Check sheet for the modelled part. Datum: model origin and axes. Units: mm. A direction names the side the tool comes from. Coordinates: 2 decimals unless noted, no trailing zeros. Write each loop counter-clockwise with the first axis right and the second up, starting at its lowest first coordinate (ties: lowest second). Pieces come first, ordered by that corner, then holes. Notation, with made-up numbers: (23.25, 1) -> (75.25, 1) arc R23 cw to (75.25, 18) -> close; hole circle Ø1 at (68.5, 22). An arc over 180 degrees is marked (long way). Put each result on its own line as item: value.
```python
from build123d import *

# Parameters (mm, degrees)
SKETCH1_W                = 25.4
SKETCH1_H                = 50.8
SKETCH1_W_2              = 19.05
SKETCH1_H_2              = 44.45
BOSS_EXTRUDE1_DEPTH      = 342.9
CUT_EXTRUDE1_DEPTH       = 1
CUT_EXTRUDE1_DEPTH_BACK  = 26.4
CUT_EXTRUDE2_REACH       = 27.4
SKETCH3_R                = 11.1125
M3_CLEARANCE_HOLE1_D     = 3.4
M3_CLEARANCE_HOLE1_DEPTH = 3.175
SKETCH9_R                = 4.5
CUT_EXTRUDE3_DEPTH       = 12.7


with BuildPart() as part:
    # Sketch1 → Boss-Extrude1 (new body, symmetric)
    with BuildSketch(Plane(origin=(0, 0, 0), x_dir=(0, 0, -1), z_dir=(1, 0, 0))):
        Rectangle(SKETCH1_W, SKETCH1_H)
        Rectangle(SKETCH1_W_2, SKETCH1_H_2, mode=Mode.SUBTRACT)
    extrude(amount=BOSS_EXTRUDE1_DEPTH, both=True)

    # Sketch2 → Cut-Extrude1 (cut, two sides)
    with BuildSketch(Plane(origin=(0, 0, -12.7), x_dir=(-1, 0, 0), z_dir=(0, 0, -1))) as cut_extrude1_sk:
        Polygon((342.9, -25.4), (342.9, 25.4), (313.570606325, -25.4), align=None)
        Polygon((-342.9, -25.4), (-313.570606325, -25.4), (-342.9, 25.4), align=None)
    extrude(amount=CUT_EXTRUDE1_DEPTH, mode=Mode.SUBTRACT)
    extrude(cut_extrude1_sk.sketch, amount=-CUT_EXTRUDE1_DEPTH_BACK, mode=Mode.SUBTRACT)

    # Sketch3 → Cut-Extrude2 (cut, up to next)
    with BuildSketch(Plane(origin=(0, 0, -12.7), x_dir=(-1, 0, 0), z_dir=(0, 0, -1)), mode=Mode.PRIVATE) as cut_extrude2_sk1:
        with Locations((-234.95, 0)):
            Circle(SKETCH3_R)
    cut_extrude2_tool1 = extrude(cut_extrude2_sk1.sketch, amount=-CUT_EXTRUDE2_REACH, mode=Mode.PRIVATE) & part.part
    add(cut_extrude2_tool1.solids().sort_by_distance((234.95, 0, -12.7))[0], mode=Mode.SUBTRACT)
    # Sketch3 → Cut-Extrude2 (cut, up to next)
    with BuildSketch(Plane(origin=(0, 0, -12.7), x_dir=(-1, 0, 0), z_dir=(0, 0, -1)), mode=Mode.PRIVATE) as cut_extrude2_sk2:
        with Locations((-190.5, 0)):
            Circle(SKETCH3_R)
    cut_extrude2_tool2 = extrude(cut_extrude2_sk2.sketch, amount=-CUT_EXTRUDE2_REACH, mode=Mode.PRIVATE) & part.part
    add(cut_extrude2_tool2.solids().sort_by_distance((190.5, 0, -12.7))[0], mode=Mode.SUBTRACT)

    # M3 Clearance Hole1
    with Locations(Plane(origin=(0, 25.4, 0), x_dir=(1, 0, 0), z_dir=(0, 1, 0))):
        with Locations((299.991366478, 0), (282.991366478, 0), (265.991366478, 0)):
            Hole(M3_CLEARANCE_HOLE1_D / 2, depth=M3_CLEARANCE_HOLE1_DEPTH)

    # Sketch9 → Cut-Extrude3 (cut)
    with BuildSketch(Plane(origin=(0, 25.4, 0), x_dir=(1, 0, 0), z_dir=(0, 1, 0))):
        with Locations((171.991366478, 0)):
            Circle(SKETCH9_R)
    extrude(amount=-CUT_EXTRUDE3_DEPTH, mode=Mode.SUBTRACT)


solid = part.part
```
Q1. Mould release check, pull along Y, two halves, no side actions. Record for faces 4 (the cylindrical face through (243.77, -6.76, -11.13)), 5 (the flat face through (5, 0, -12.7)), 6 (the flat face through (4, -25.4, 0)): released by +Y, released by -Y, zero draft, split by the parting line, or undercut.
Recorded:
face 4: undercut
face 5: zero draft
face 6: released by -Y
Q2. Tool access check on faces 1 (the flat face through (5, 0, -9.525)), 2 (the flat face through (-328.304, 0.119, -10.407)), 3 (the cylindrical face through (199.32, -6.76, -11.13)). Record the directions out of +Z, -Z, +X, -X, +Y, -Y that give a thin tool (end or side, any length) a straight path to the whole face; none if there is none.
Recorded:
face 1: +X, -X
face 2: +Z, -Z, -X, -Y
face 3: -Z
Q3. Depth check by flat-ended pin: P1, Ø13.5, axis at x = 190.5, y = 0, coming from the -Z side (3 decimals); P2, Ø12, axis at y = 2, z = -8, coming from the -X side; P3, Ø2.5, axis at x = 265.99, z = 0, coming from the +Y side (3 decimals). Enter the tip coordinate at first touch or a pass-through.
Recorded:
P1: stops at z = 9.525
P2: stops at x = -332.74
P3: stops at y = -22.225
Q4. Material ranges on line 1 along Z through (x, y) = (-157, 12.5) (3 decimals); line 2 along Y through (x, z) = (200.5, 2.5) (3 decimals); line 3 along Y through (x, z) = (190.5, -10.55), recorded low to high.
Recorded:
line 1: z = -12.7 to -9.525, 9.525 to 12.7
line 2: y = -25.4 to -22.225, 22.225 to 25.4
line 3: y = -25.4 to -11.11, 11.11 to 25.4
Q5. Cross-section at B-B (y = 0). Record the cut outline in (x, z) (1 decimal), plus the area to 3 significant figures.
Recorded:
outline: (-328.2, -12.7) -> (179.4, -12.7) -> (179.4, -9.5) -> (-328.2, -9.5) -> close; (-328.2, 9.5) -> (328.2, 9.5) -> (328.2, 12.7) -> (-328.2, 12.7) -> close; (201.6, -12.7) -> (223.8, -12.7) -> (223.8, -9.5) -> (201.6, -9.5) -> close; (246.1, -12.7) -> (328.2, -12.7) -> (328.2, -9.5) -> (246.1, -9.5) -> close
area: 4,030 mm2
Q6. Cross-section at C-C (x = 190.5). Record the cut outline in (y, z) (1 decimal), plus the area to 3 significant figures.
Recorded:
outline: (-25.4, -12.7) -> (-11.1, -12.7) -> (-11.1, -9.5) -> (-22.2, -9.5) -> (-22.2, 9.5) -> (22.2, 9.5) -> (22.2, -9.5) -> (11.1, -9.5) -> (11.1, -12.7) -> (25.4, -12.7) -> (25.4, 12.7) -> (-25.4, 12.7) -> close
area: 373 mm2
Q7. Cross-section at A-A (x = -80). Record the cut outline in (y, z) (3 decimals).
Recorded:
outline: (-25.4, -12.7) -> (25.4, -12.7) -> (25.4, 12.7) -> (-25.4, 12.7) -> close; hole (-22.225, -9.525) -> (22.225, -9.525) -> (22.225, 9.525) -> (-22.225, 9.525) -> close
